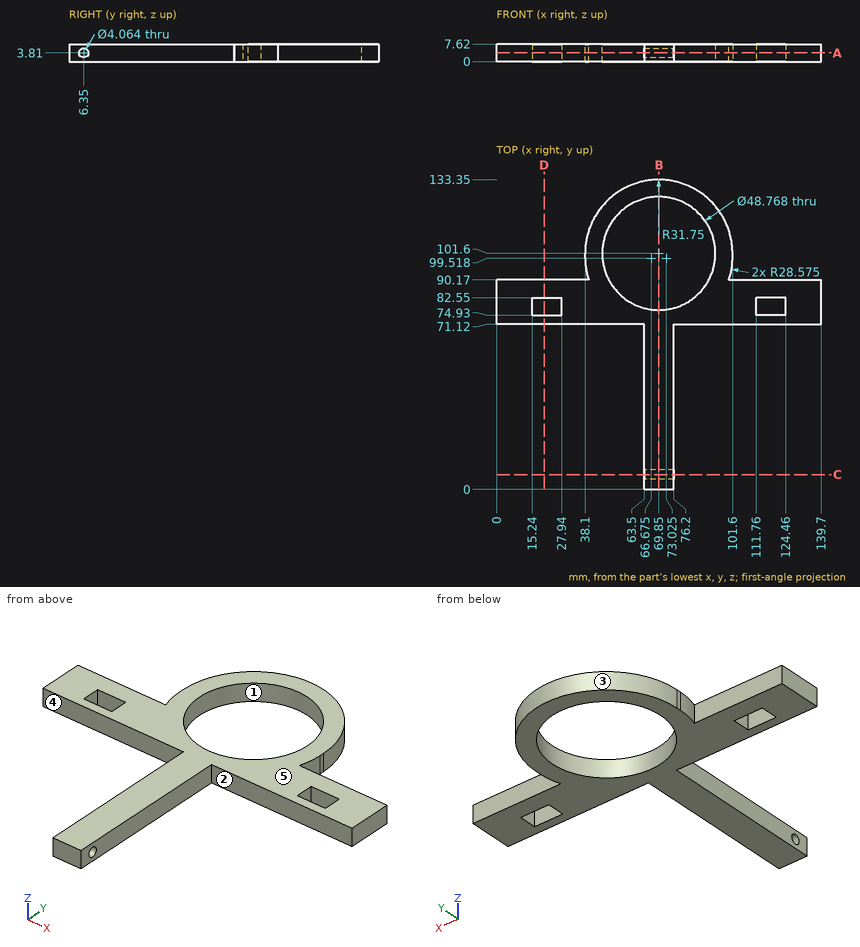
Geometry check sheet. Reference: drawing and pictorial views, mm from the part's lowest x, y, z. A direction names the side the tool comes from. Round coordinates to 2 decimals unless told otherwise and drop trailing zeros. Loops run counter-clockwise (first coordinate to the right, second up) from the corner with the lowest first, then second, coordinate; pieces in that order, holes last. Notation, with made-up numbers: (49.25, 12) - (82.25, 12) arc R13 ccw to (82.25, 33) - close; hole circle Ø10 at (66, 57). An arc over 180 degrees is marked (long way). One line per question, with ' | ' between items. Start each with the question number.
1. Depth check by flat-ended pin: pin 1 (3.5 mm diameter, centred on y = 6.35, z = 3.81, fed in from -X); pin 2 (2.5 mm diameter, centred on x = 116, z = 4, fed in from +Y); pin 3 (1 mm diameter, centred on x = 46, y = 118.5, fed in from -Z); pin 4 (1 mm diameter, centred on y = 100.5, z = 3.5, fed in from -X). Enter the tip coordinate at first touch or a pass-through.
2. Cross-section at C-C on y = 6.35. Record the cut outline in (x, z).
3. Cross-section at D-D on x = 20.5. Record the cut outline in (y, z).
4. Scan lines: line 1 (X direction, y = 76, z = 6.75); line 2 (Y direction, x = 69, z = 3.81); line 3 (Y direction, x = 69.5, z = 7). Record each from-to range of solid material in increasing order. Write a range as [from, to].
5. Tool access check on the marked faces 4 and 5. Record the directions out of +Z, -Z, +X, -X, +Y, -Y that give a thin tool (end or side, any length) a straight path to the whole face; none if there is none.
6. Cross-section at A-A on z = 3.81. Record the cut outline in (x, y) (3 decimals).
7. Draft check along X on the marked faces 1, 2 and 3. Enter one of: released by +X, released by -X, zero draft, split by the parting line, or undercut.
8. Cross-section at B-B on x = 69.85. Record the cut outline in (y, z), then the cut area to 3 significant figures.
Taken from the geometry:
1) pin 1: through | pin 2: y = 90.17 | pin 3: z = 0 | pin 4: x = 38.1
2) outline: (63.5, 0) - (76.2, 0) - (76.2, 1.78) - (63.5, 1.78) - close; (63.5, 5.84) - (76.2, 5.84) - (76.2, 7.62) - (63.5, 7.62) - close
3) outline: (71.12, 0) - (74.93, 0) - (74.93, 7.62) - (71.12, 7.62) - close; (82.55, 0) - (90.17, 0) - (90.17, 7.62) - (82.55, 7.62) - close
4) line 1: [0, 15.24], [27.94, 111.76], [124.46, 139.7] | line 2: [0, 4.32], [8.38, 77.23], [125.97, 133.34] | line 3: [0, 77.22], [125.98, 133.35]
5) face 4: +Z, -Z, -X, -Y | face 5: +Z, +X, -X, +Y, -Y
6) outline: (0, 71.12) - (63.5, 71.12) - (63.5, 8.382) - (76.2, 8.382) - (76.2, 71.12) - (139.7, 71.12) - (139.7, 90.17) - (100.028, 90.17) arc R28.575 ccw to (101.6, 99.518) - (101.6, 101.6) arc R31.75 ccw to (38.1, 101.6) - (38.1, 99.518) arc R28.575 ccw to (39.672, 90.17) - (0, 90.17) - close; (63.5, 0) - (76.2, 0) - (76.2, 4.318) - (63.5, 4.318) - close; hole (15.24, 74.93) - (27.94, 74.93) - (27.94, 82.55) - (15.24, 82.55) - close; hole circle Ø48.768 at (69.85, 101.6); hole (111.76, 74.93) - (124.46, 74.93) - (124.46, 82.55) - (111.76, 82.55) - close
7) face 1: undercut | face 2: zero draft | face 3: split by the parting line
8) outline: (0, 0) - (77.22, 0) - (77.22, 7.62) - (0, 7.62) - close; (125.98, 0) - (133.35, 0) - (133.35, 7.62) - (125.98, 7.62) - close; hole circle Ø4.06 at (6.35, 3.81) | area: 632 mm²
